```python
from build123d import *

# Parameters (mm, degrees)
F0_W     = 25.4
F0_H     = 25.4
F1_DEPTH = 5.08
F3_DEPTH = 1.524


with BuildPart() as f1:
    # F0 (on Front) → F1 (new body)
    with BuildSketch(Plane.XZ):
        Rectangle(F0_W, F0_H)
    extrude(amount=F1_DEPTH)

    # F2 (on face) → F3 (join)
    with BuildSketch(Plane.XZ.offset(5.08)):
        Polygon((-3.770767, 10.104783), (-11.998158, 2.208696), (-11.499409, 1.213393), (-6.533915, 5.693889), (-7.137069, 1.319007), (1.363335, 7.181271), (2.750369, 1.142781), (8.985079, 8.0043), (11.209368, 3.565513), (12.137308, 4.030507), (9.09347, 10.104783), (3.907741, 4.030507), (3.459665, 10.104783), (-4.764671, 4.030507), align=None)
        Polygon((-3.500791, -2.970403), (-11.84413, -8.724348), (-11.954566, -10.380869), (-5.715, -6.846956), (-6.101522, -11.264347), (2.750369, -5.442571), (2.750369, -10.549271), (9.664643, -5.442571), (11.623261, -8.282608), (12.397479, -7.083917), (9.359348, -2.970403), (3.83674, -8.08217), (3.459665, -2.970403), (-4.764671, -8.669131), align=None)
    extrude(amount=F3_DEPTH)


solid = f1.part
```
Build history of the part. All positions in model axes, mm. A direction names the side the tool comes from. Coordinates: 2 decimals unless noted, no trailing zeros. Order: outer loops, then holes, each group sorted by start corner. A loop starts at its lowest first (then second) coordinate and runs counter-clockwise, first axis right, second up. Notation, with made-up numbers: (26, 10) -> (54, 10) arc R19 ccw to (54, 25) -> close; hole circle Ø8 at (89, 55.5). An arc over 180 degrees is marked (long way). Answer in a Markdown table with one row per item. Add a question column.
Q1. Band-saw the part on A-A, the plane z = -10. List the corners of the cut face in (x, y), then the cut area to 3 significant figures.
Q2. Band-saw the part on C-C, the plane x = 7.5. List the corners of the cut face in (y, z).
Q3. Drop a flat-ended pin along its axis: pin 1 (1.7 mm diameter, centred on y = -6, z = -8, fed in from -X). Give the stop position or say it passes through.
Q4. Band-saw the part on D-D, the plane z = -4.25. List the corners of the cut face in (x, y), then the cut area to 3 significant figures.
Q5. Band-saw the part on B-B, the plane x = -3. List the corners of the cut face in (y, z), then the cut area to 3 significant figures.
Q6. Mould opens along Z. For faces 4 (the face through (-7.83, -5.83, 6.21)), 5 (the face through (-9.051, -5.831, 3.422)), 6 (the face through (-1, -6.604, 6)) say: +Z half, -Z half, draft (parallel to the pull), parting line (faces both ways), or undercut.
Q7. Wall check: line 1 along X through (y, z) = (-5.5, -9); line 2 along Y through (x, z) = (-8.75, -8.75); line 3 along Z through (x, y) = (-3, -5.5). Give the ranges that are in metal, low to high. Write a range as [from, to].
Q8. Which spindle directions (+Z, -Z, +X, -X, +Y, -Y) get a long thin tool onto all of the face, cutting with end or side? Do faces 1 (the face through (3.687, -5.831, 7.025)), 2 (the face through (-2.946, -5.831, 4.209)), 3 (the face through (11.667, -5.831, 3.795)). Say none if no direction does.
Answers follow:
| question | item | result |
|---|---|---|
| 1 | outline | (-12.7, -5.08) -> (-11.93, -5.08) -> (-11.93, -6.6) -> (-11.28, -6.6) -> (-11.28, -5.08) -> (-5.99, -5.08) -> (-5.99, -6.6) -> (-4.18, -6.6) -> (-4.18, -5.08) -> (2.75, -5.08) -> (2.75, -6.6) -> (3.49, -6.6) -> (3.49, -5.08) -> (12.7, -5.08) -> (12.7, 0) -> (-12.7, 0) -> close |
| 1 | area | 134 mm^2 |
| 2 | outline | (-6.6, -7.04) -> (-5.08, -7.04) -> (-5.08, -12.7) -> (0, -12.7) -> (0, 12.7) -> (-5.08, 12.7) -> (-5.08, 8.24) -> (-6.6, 8.24) -> (-6.6, 6.37) -> (-5.08, 6.37) -> (-5.08, -4.69) -> (-6.6, -4.69) -> close |
| 3 | pin 1 | x = -11.85 |
| 4 | outline | (-12.7, -5.08) -> (-5.36, -5.08) -> (-5.36, -6.6) -> (-3.78, -6.6) -> (-3.78, -5.08) -> (1.61, -5.08) -> (1.61, -6.6) -> (3.55, -6.6) -> (3.55, -5.08) -> (7.98, -5.08) -> (7.98, -6.6) -> (10.3, -6.6) -> (10.3, -5.08) -> (12.7, -5.08) -> (12.7, 0) -> (-12.7, 0) -> close |
| 4 | area | 138 mm^2 |
| 5 | outline | (-6.6, -9.22) -> (-5.08, -9.22) -> (-5.08, -12.7) -> (0, -12.7) -> (0, 12.7) -> (-5.08, 12.7) -> (-5.08, 5.33) -> (-6.6, 5.33) -> (-6.6, 4.17) -> (-5.08, 4.17) -> (-5.08, -7.45) -> (-6.6, -7.45) -> close |
| 5 | area | 134 mm^2 |
| 6 | face 4 | +Z half |
| 6 | face 5 | undercut |
| 6 | face 6 | draft |
| 7 | line 1 | [-11.86, -9.52], [-5.9, -2.66], [2.75, 4.85] |
| 7 | line 2 | [-5.08, 0] |
| 7 | line 3 | [-9.22, -7.45], [4.17, 5.33] |
| 8 | face 1 | +Z, -Y |
| 8 | face 2 | -Y |
| 8 | face 3 | +X, -Y |
